Geometry: final body of the model. Coordinates: model frame, mm. A direction names the side the tool comes from. Give positions to 0.01 mm unless a question says otherwise; leave off trailing zeros. Write each loop counter-clockwise with the first axis right and the second up, starting at its lowest first coordinate (ties: lowest second). Pieces come first, ordered by that corner, then holes.
from build123d import *

# Parameters (mm, degrees)
F0_R     = 14.5
F1_DEPTH = 3
F2_W     = 4
F2_H     = 30
F3_DEPTH = 1.5
F4_R     = 5
F4_R_2   = 3
F5_DEPTH = 1.5
F6_R     = 3
F7_DEPTH = 1.5
F8_R     = 1
F9_DEPTH = 1.5
F10_SIZE = 1


with BuildPart() as f1:
    # F0 (on Top) → F1 (new body)
    with BuildSketch(Plane.XY):
        Circle(F0_R)
    extrude(amount=F1_DEPTH)

    # F2 (on face) → F3 (cut)
    with BuildSketch(Plane.XY.offset(3)):
        Rectangle(F2_W, F2_H)
    extrude(amount=-F3_DEPTH, mode=Mode.SUBTRACT)

    # F4 (on face) → F5 (cut)
    with BuildSketch(Plane.XY.offset(3)):
        Circle(F4_R)
        Circle(F4_R_2, mode=Mode.SUBTRACT)
    extrude(amount=-F5_DEPTH, mode=Mode.SUBTRACT)

    # F6 (on face) → F7 (join)
    with BuildSketch(Plane.XY.offset(3)):
        Circle(F6_R)
    extrude(amount=-F7_DEPTH)

    # F8 (on face) → F9 (cut)
    with BuildSketch(Plane.XY.offset(3)):
        with Locations((10, 0)):
            Circle(F8_R)
        with Locations((-10, 0)):
            Circle(F8_R)
    extrude(amount=-F9_DEPTH, mode=Mode.SUBTRACT)

    # F10
    f10_edges = [f1.edges().sort_by_distance(p)[0] for p in [
        (-14.5, 0, 0),
    ]]
    chamfer(f10_edges, length=F10_SIZE)


solid = f1.part
Q1. Ray query, line 1 along Z through (x, y) = (-1.5, 7); line 2 along X through (y, z) = (-6, 2.7); line 3 along X through (y, z) = (10.5, 1.8). Return the intervals inside material, ascending.
Filled sheet:
line 1: z = 0 to 1.5
line 2: x = -13.2 to -2, 2 to 13.2
line 3: x = -10 to -2, 2 to 10
Q2. Section A-A on y = 0. Output: boundary loops of the cut face in (x, z).
Filled sheet:
outline: (-14.5, 1) - (-13.5, 0) - (13.5, 0) - (14.5, 1) - (14.5, 3) - (11, 3) - (11, 1.5) - (9, 1.5) - (9, 3) - (5, 3) - (5, 1.5) - (3, 1.5) - (3, 3) - (-3, 3) - (-3, 1.5) - (-5, 1.5) - (-5, 3) - (-9, 3) - (-9, 1.5) - (-11, 1.5) - (-11, 3) - (-14.5, 3) - close
Q3. Pull-direction query (Y, two-part tool) for faces 1 (the flat face through (0, 0, 0)), 2 (the cylindrical face through (6.691, -12.864, 1.986)), 3 (the cylindrical face through (-5, 0, 2)); classes: released by +Y, released by -Y, zero draft, split by the parting line, or undercut.
Filled sheet:
face 1: zero draft
face 2: split by the parting line
face 3: undercut
Q4. Pin query (flat end, axial travel): P1, Ø1, axis at x = 10, y = 0, coming from the +Z side; P2, Ø1.2, axis at y = 7.5, z = 2, coming from the +X side; P3, Ø2.5, axis at x = -10, y = 0, coming from the -Z side; P4, Ø1.5, axis at x = 3.5, z = 2.5, coming from the -Y side. Return the tip coordinate at first contact, or that it passes through.
Filled sheet:
P1: stops at z = 1.5
P2: stops at x = 12.75
P3: stops at z = 0
P4: stops at y = -14.24
Q5. Access query for faces 4 (the flat face through (2, -10, 2)), 5 (the cylindrical face through (5, 0, 2)), 6 (the flat face through (2, 9, 2)). Directions: +Z, -Z, +X, -X, +Y, -Y. A direction counts if a zero-diameter tool reaches every point of the face in a straight line with its end or side. Return the directions, or none.
Filled sheet:
face 4: +Z, -Y
face 5: +Z
face 6: +Z, +Y
Q6. Section B-B on x = 0. Output: boundary loops of the cut face in (y, z).
Filled sheet:
outline: (-14.5, 1) - (-13.5, 0) - (13.5, 0) - (14.5, 1) - (14.5, 1.5) - (3, 1.5) - (3, 3) - (-3, 3) - (-3, 1.5) - (-14.5, 1.5) - close
